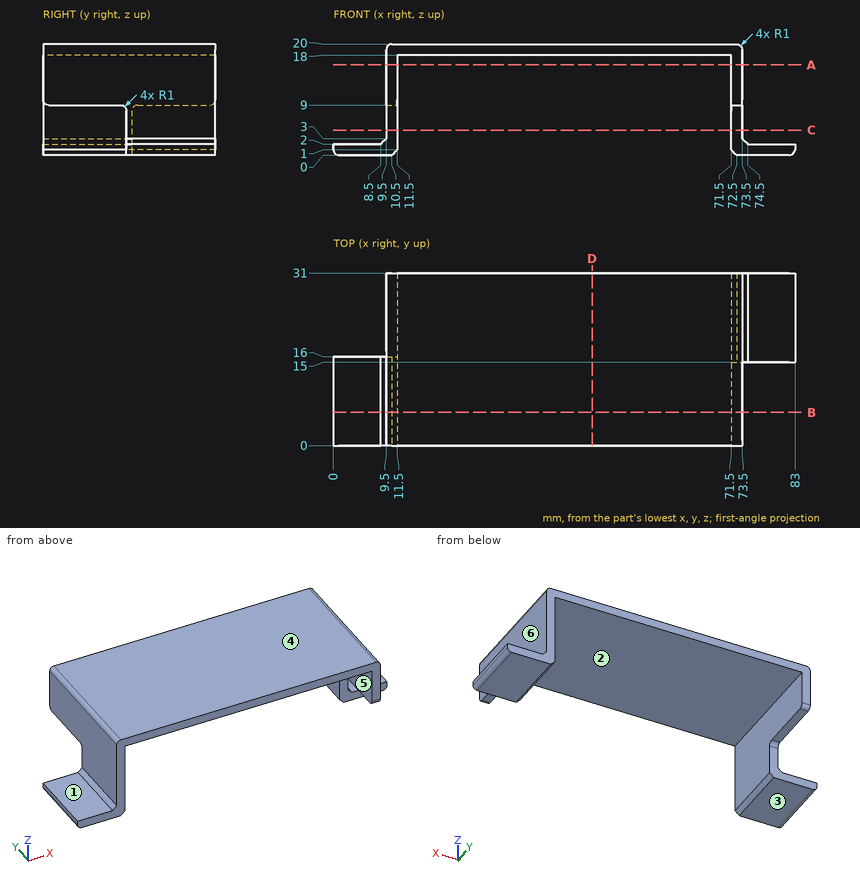
Design review of the part shown in the three views and the two pictorial views. Dimensions are in mm from the part's minimum x, y and z. A direction names the side the tool comes from. Give positions to 0.01 mm unless a question says otherwise; leave off trailing zeros. Write each loop counter-clockwise with the first axis right and the second up, starting at its lowest first coordinate (ties: lowest second). Pieces come first, ordered by that corner, then holes. Notation, with made-up numbers: M 79,69 L 131,69 A30 ccw 131,101 Z; hole C 37.5,77.5 d4. An arc over 180 degrees is marked long. Answer as CSV lines item,"result".
1. Draft analysis for pull direction X (two halves, no side actions). For the marked faces 4, 5 and 6, state which applies: +X half, -X half, draft (parallel to the pull), parting line (faces both ways), or undercut.
Findings:
face 4,"draft"
face 5,"undercut"
face 6,"+X half"
2. Consider section D-D, the plane x = 46.5. Write out the cut boundary in (y, z).
Findings:
outline,"M 0,18 L 31,18 L 31,20 L 0,20 Z"
3. Consider section B-B, the plane y = 6. Write out the cut boundary in (x, z).
Findings:
outline,"M 0,1 A1 ccw 1,0 L 10.5,0 L 11.5,1 L 11.5,18 L 71.5,18 L 71.5,9 L 73.5,9 L 73.5,19 A1 ccw 72.5,20 L 10.5,20 A1 ccw 9.5,19 L 9.5,3 L 8.5,2 L 0,2 Z"
4. Consider section A-A, the plane z = 16.25. Write out the cut boundary in (x, y).
Findings:
outline,"M 9.5,0 L 11.5,0 L 11.5,31 L 9.5,31 Z; M 71.5,0 L 73.5,0 L 73.5,31 L 71.5,31 Z"
5. For pin 1 (2 mm diameter, centred on x = 10.5, y = 20.5, fed in from -Z); pin 2 (10 mm diameter, centred on y = 10, z = 9.5, fed in from +X); pin 3 (4 mm diameter, centred on y = 20, z = 9, fed in from -X); pin 4 (4 mm diameter, centred on x = 49.5, z = 15, fed in from -Y), all flat-tipped, find the tip position at first contact; note any pin that passes through.
Findings:
pin 1,"stops at z = 9"
pin 2,"stops at x = 73.5"
pin 3,"stops at x = 9.5"
pin 4,"passes through"
6. Wall thickness on line 1 (X direction, y = 15, z = 9.75); line 2 (Z direction, x = 38.5, y = 16.5); line 3 (Y direction, x = 10.5, z = 3): over which ranges is each line inside the solid? List them lowest first.
Findings:
line 1,"x = 9.5 to 11.5, 71.5 to 73.5"
line 2,"z = 18 to 20"
line 3,"y = 0 to 16"
7. For the marked faces 1, 2 and 3, list the 3-axis set-ups (+Z, -Z, +X, -X, +Y, -Y) from which the entire face can be reached by the end or side of a thin tool; tool diameter is ignored.
Findings:
face 1,"+Z, -X, +Y, -Y"
face 2,"-Z, +Y, -Y"
face 3,"-Z, +X, -X, +Y, -Y"
8. Consider section C-C, the plane z = 4.5. Write out the cut boundary in (x, y).
Findings:
outline,"M 9.5,0 L 11.5,0 L 11.5,16 L 9.5,16 Z; M 71.5,15 L 73.5,15 L 73.5,31 L 71.5,31 Z"
